Input: part model. Units: mm. Frame: model coordinates. A direction names the side the tool comes from. Round coordinates to 2 decimals unless told otherwise and drop trailing zeros. Order: outer loops, then holes, each group sorted by start corner. A loop starts at its lowest first (then second) coordinate and runs counter-clockwise, first axis right, second up.
Item 1: Reachability of faces 4 (the flat face through (513, -10, 12)), 5 (the flat face through (513, -9, 0)) from +Z, -Z, +X, -X, +Y, -Y: full face, straight path, thin tool, end or side. Return the list, or none.
Item 2: Cut plane B-B on z = 19.25. Output: boundary loops of the cut face in (x, y), then the cut area to 3 significant figures.
Item 3: Line query: L1, parallel to Y at x = 259, z = 6.75; L2, parallel to X at y = -15.5, z = 2.5. Output: solid intervals per line, ascending.
Item 4: Cut plane A-A on x = 440.5. Output: boundary loops of the cut face in (y, z).
Item 5: Cut plane C-C on y = -16.5. Output: boundary loops of the cut face in (x, z), then the cut area to 3 significant figures.
Item 6: Mould query, pull axis X, two halves, no side actions, for faces 1 (the flat face through (1040, -17, 12)), 2 (the flat face through (513, -25, 12)), 3 (the flat face through (513, -9, 25)). Classes: released by +X, released by -X, zero draft, split by the parting line, or undercut.
```python
from build123d import *

# Parameters (mm, degrees)
F0_W     = 1040
F0_H     = 25
F1_DEPTH = 35
F2_W     = 1000
F2_H     = 15
F3_DEPTH = 25.001


with BuildPart() as f1:
    # F0 (on Front) → F1 (new body)
    with BuildSketch(Plane.XZ):
        with Locations((520, 12.5)):
            Rectangle(F0_W, F0_H)
    extrude(amount=F1_DEPTH)

    # F2 (on face) → F3 (cut, through all)
    with BuildSketch(Plane(origin=(0, 0, 0), x_dir=(1, 0, 0), z_dir=(0, 0, -1))):
        with Locations((520, 17.5)):
            Rectangle(F2_W, F2_H)
    extrude(amount=-F3_DEPTH, mode=Mode.SUBTRACT)


solid = f1.part
```
From the geometry:
1. face 4: +Z, -Z
1. face 5: -Z, +X, -X, +Y, -Y
2. outline: (0, -35) - (1040, -35) - (1040, 0) - (0, 0) - close; hole (20, -25) - (1020, -25) - (1020, -10) - (20, -10) - close
2. area: 21,400 mm2
3. L1: y = -35 to -25, -10 to 0
3. L2: x = 0 to 20, 1020 to 1040
4. outline: (-35, 0) - (-25, 0) - (-25, 25) - (-35, 25) - close; (-10, 0) - (0, 0) - (0, 25) - (-10, 25) - close
5. outline: (0, 0) - (20, 0) - (20, 25) - (0, 25) - close; (1020, 0) - (1040, 0) - (1040, 25) - (1020, 25) - close
5. area: 1,000 mm2
6. face 1: released by +X
6. face 2: undercut
6. face 3: zero draft
